Model file for the job. Use its own axes, mm. A direction names the side the tool comes from. Coordinates: 2 decimals unless noted, no trailing zeros. Write each loop counter-clockwise with the first axis right and the second up, starting at its lowest first coordinate (ties: lowest second). Pieces come first, ordered by that corner, then holes. Notation, with made-up numbers: (22, 34.5) - (52, 34.5) arc R21 ccw to (52, 55.5) - close; hole circle Ø7 at (67.5, 56.5). An arc over 180 degrees is marked (long way). Put each result on its own line as item: value. Start each with the question number.
1. Saw through at D-D, the plane z = 1.5. Write the cut outline in (x, y).
2. Drill centre lines: L1, parallel to Z at x = 52.5, y = 7.5; L2, parallel to X at y = -0.75, z = -8.5; L3, parallel to Z at x = 2, y = 5.5. Where is each one in solid material? Low to high. Write a range as from..to.
3. Saw through at A-A, the plane y = 1.75. Write the cut outline in (x, z), plus the area to 3 significant figures.
4. Which spindle directions (+Z, -Z, +X, -X, +Y, -Y) get a long thin tool onto all of the face, cutting with end or side? Do faces 1 (the face through (-10, 0, 20.538)), 2 (the face through (52.902, 0, -10)), 3 (the face through (38.539, -7.395, 5.857)). Say none if no direction does.
5. Saw through at B-B, the plane z = 14. Write the cut outline in (x, y).
6. Saw through at C-C, the plane y = -10. Write the cut outline in (x, z).
7. Drop flat-ended pins along their axis: P1, Ø2, axis at x = 59.5, z = 6, coming from the -Y side; P2, Ø1, axis at x = 6.5, y = 6, coming from the +Z side; P3, Ø6, axis at y = 10, z = 31, coming from the +X side. Give the stop position or say it passes through.
```python
from build123d import *

# Parameters (mm, degrees)
F1_DEPTH = 15
F2_DEPTH = 15
F3_DEPTH = 15


with BuildPart() as f1:
    # F0 (on Front) → F1 (new body)
    with BuildSketch(Plane.XZ):
        with BuildLine():
            Line((-52.9015958309, 20.53822577), (-52.9015958309, -20.53822577))
            Line((-52.9015958309, -20.53822577), (52.9015958309, -20.53822577))
            Line((52.9015958309, -20.53822577), (52.9015958309, 0))
            ThreePointArc((52.9015958309, 0), (38.3788771154, 6.0155070545), (32.3633700609, 20.53822577))
            Line((32.3633700609, 20.53822577), (-52.9015958309, 20.53822577))
        make_face()
    extrude(amount=-F1_DEPTH)

    # F2 (add): a face of the model
    f2_faces = [f1.faces().sort_by_distance(p)[0] for p in [
        (-3.6461449369, 0, -0.9755146466),
    ]]
    extrude(f2_faces, amount=F2_DEPTH)

    # F0 (on Front) → F3 (join)
    with BuildSketch(Plane.XZ):
        with BuildLine():
            Line((52.9015958309, 11.3889886989), (52.9015958309, 0))
            ThreePointArc((52.9015958309, 0), (67.4243145464, 6.0155070545), (73.4398216009, 20.53822577))
            ThreePointArc((73.4398216009, 20.53822577), (52.9015958309, 41.07645154), (32.3633700609, 20.53822577))
            Line((32.3633700609, 20.53822577), (43.7523587598, 20.53822577))
            ThreePointArc((43.7523587598, 20.53822577), (52.9015958309, 29.6874628411), (62.050832902, 20.53822577))
            ThreePointArc((62.050832902, 20.53822577), (59.3710834066, 14.0687381943), (52.9015958309, 11.3889886989))
        make_face()
        with BuildLine():
            ThreePointArc((32.3633700609, 20.53822577), (38.3788771154, 6.0155070545), (52.9015958309, 0))
            Line((52.9015958309, 0), (52.9015958309, 11.3889886989))
            ThreePointArc((52.9015958309, 11.3889886989), (46.4321082553, 14.0687381943), (43.7523587598, 20.53822577))
            Line((43.7523587598, 20.53822577), (32.3633700609, 20.53822577))
        make_face()
    extrude(amount=-F3_DEPTH)


solid = f1.part
```
Final values:
1. outline: (-52.9, -15) - (45.2, -15) - (45.2, 0) - (60.61, 0) - (60.61, 15) - (-52.9, 15) - close
2. L1: z = -20.54..11.4, 29.68..41.07
2. L2: x = -52.9..52.9
2. L3: z = -20.54..20.54
3. outline: (-52.9, -20.54) - (52.9, -20.54) - (52.9, 0) arc R20.54 ccw (long way) to (32.36, 20.54) - (-52.9, 20.54) - close; hole circle Ø18.3 at (52.9, 20.54)
3. area: 5,080 mm²
4. face 1: +Z, -X, +Y, -Y
4. face 2: -Z, +X, +Y, -Y
4. face 3: +Z, +X, -Y
5. outline: (-52.9, -15) - (33.43, -15) - (33.43, 0) - (46.5, 0) - (46.5, 15) - (-52.9, 15) - close; (59.3, 0) - (72.37, 0) - (72.37, 15) - (59.3, 15) - close
6. outline: (-52.9, -20.54) - (52.9, -20.54) - (52.9, 0) arc R20.54 cw to (32.36, 20.54) - (-52.9, 20.54) - close
7. P1: stops at y = 0
7. P2: stops at z = 20.54
7. P3: stops at x = 72.04
